The listing builds one solid part. Answer for the finished solid, in the listing's coordinates (mm). A direction names the side the tool comes from. Give positions to 0.01 mm unless a question says otherwise; leave off trailing zeros. Order: outer loops, then holes, each group sorted by start corner. A loop starts at its lowest first (then second) coordinate and runs counter-clockwise, first axis right, second up. Notation, with made-up numbers: (1.5, 26) - (58.5, 26) arc R33 cw to (58.5, 63) - close; hole circle Ø2 at (80, -24.75). An arc over 180 degrees is marked (long way). Answer in a Markdown table with one row per item.
Autodesk Inventor part; units mm, degrees
ref_plane "YZ Plane" through (0, 0, 0) normal (1, 0, 0) x (0, 1, 0)
ref_plane "XZ Plane" through (0, 0, 0) normal (0, 1, 0) x (-1, 0, 0)
ref_plane "XY Plane" through (0, 0, 0) normal (0, 0, 1) x (1, 0, 0)
sketch "Boceto1" plane through (0, 0, 0) normal (0, 0, 1) x (1, 0, 0)
  line L0 (-15, 15) -> (15, 15)
  line L1 (15, 15) -> (15, -15)
  line L2 (15, -15) -> (-15, -15)
  line L3 (-15, -15) -> (-15, 15)
  line L4 (-15, 15) -> (15, -15) construction
  line L5 (15, 15) -> (-15, -15) construction
  line L6 (-12.5, 12.5) -> (12.5, 12.5)
  line L7 (12.5, 12.5) -> (12.5, -12.5)
  line L8 (12.5, -12.5) -> (-12.5, -12.5)
  line L9 (-12.5, -12.5) -> (-12.5, 12.5)
  line L10 (-12.5, 12.5) -> (12.5, -12.5) construction
  line L11 (12.5, 12.5) -> (-12.5, -12.5) construction
  point P0 (0, 0)
  dimension "d2" = 30
  dimension "d3" = 30
  dimension "d4" = 25
  dimension "d5" = 25
extrude "Extrusión1" add sketch "Boceto1" against normal mid plane 480
properties part number "Barra_480" material "Acero"
Item 1: Find section A-A on z = 107. Write down the section's boundary in (x, y).
Answer block:
| item | result |
|---|---|
| outline | (-15, -15) - (15, -15) - (15, 15) - (-15, 15) - close; hole (-12.5, -12.5) - (12.5, -12.5) - (12.5, 12.5) - (-12.5, 12.5) - close |
Item 2: Which of the six approach directions +Z, -Z, +X, -X, +Y, -Y give full straight-line access (tool end or side, diameter ignored) to faces 4 (the face through (-14, 0, 240)), 5 (the face through (0, 12.5, 3))?
Answer block:
| item | result |
|---|---|
| face 4 | +Z, +X, -X, +Y, -Y |
| face 5 | +Z, -Z |
Item 3: Find section B-B on x = -8.5. Write down the section's boundary in (y, z).
Answer block:
| item | result |
|---|---|
| outline | (-15, -240) - (-12.5, -240) - (-12.5, 240) - (-15, 240) - close; (12.5, -240) - (15, -240) - (15, 240) - (12.5, 240) - close |
Item 4: Consider line 1 (Y direction, x = 11.5, z = -171). Determine where the line is inside the solid, lowest interval first.
Answer block:
| item | result |
|---|---|
| line 1 | -15 to -12.5, 12.5 to 15 |
Item 5: Determine the mould class of faces 1 (the face through (15, 0, 3)), 2 (the face through (-14, 0, -240)), 3 (the face through (-12.5, 0, 3)) for opening direction X: pulls with the +X half, pulls with the -X half, needs draft (parallel to the pull), parting line crosses it, or undercut.
Answer block:
| item | result |
|---|---|
| face 1 | pulls with the +X half |
| face 2 | needs draft |
| face 3 | undercut |
Item 6: This flat-tipped pin is pushed along its axis until it touches: P1, Ø10, axis at x = -11, y = -11.5, coming from the -Z side. Where does it stop, or does it pass through?
Answer block:
| item | result |
|---|---|
| P1 | z = -240 |
